Part model, mm, in its own coordinate system. A direction names the side the tool comes from. Coordinates: 2 decimals unless noted, no trailing zeros. Loops run counter-clockwise (first coordinate to the right, second up) from the corner with the lowest first, then second, coordinate; pieces in that order, holes last. Notation, with made-up numbers: (87.25, 12) -> (131.25, 12) arc R22 cw to (131.25, 21) -> close; hole circle Ø8 at (-16, 66). An arc over 180 degrees is marked (long way). One line per item, written item: value. Start each with the question number.
from build123d import *

# Parameters (mm, degrees)
F0_W     = 5.9
F0_H     = 0.3
F1_DEPTH = 2.5
F0_H_2   = 3.125
F2_DEPTH = 0.2
F4_DEPTH = 6.501


with BuildPart() as f1:
    # F0 (on Front) → F1 (new body)
    with BuildSketch(Plane.XZ):
        Polygon((-3.25, 16.5), (-3.25, 0), (-2.95, 0), (-2.95, 1), (-2.95, 1.3), (-2.95, 4.425), (-2.95, 4.725), (-2.95, 7.85), (-2.95, 8.15), (-2.95, 11.275), (-2.95, 11.575), (-2.95, 14.7), (-2.95, 15), (-2.95, 16.5), align=None)
        Polygon((2.95, 1), (2.95, 0), (3.25, 0), (3.25, 16.5), (2.95, 16.5), (2.95, 15), (2.95, 14.7), (2.95, 11.575), (2.95, 11.275), (2.95, 8.15), (2.95, 7.85), (2.95, 4.725), (2.95, 4.425), (2.95, 1.3), align=None)
        with Locations((0, 14.85)):
            Rectangle(F0_W, F0_H)
        with Locations((0, 11.425)):
            Rectangle(F0_W, F0_H)
        with Locations((0, 8)):
            Rectangle(F0_W, F0_H)
        with Locations((0, 4.575)):
            Rectangle(F0_W, F0_H)
        with Locations((0, 1.15)):
            Rectangle(F0_W, F0_H)
    extrude(amount=F1_DEPTH)

    # F0 (on Front) → F2 (join)
    with BuildSketch(Plane.XZ):
        with Locations((0, 13.1375)):
            Rectangle(F0_W, F0_H_2)
        with Locations((0, 6.2875)):
            Rectangle(F0_W, F0_H_2)
    extrude(amount=F2_DEPTH)

    # F3 (on face) → F4 (cut, through all)
    with BuildSketch(Plane.YZ.offset(3.25)):
        Polygon((-1.9, 0), (-0.6, 0), (-0.6, 1), (-1.25, 1), align=None)
    extrude(amount=-F4_DEPTH, mode=Mode.SUBTRACT)


solid = f1.part
1) Pull direction X, two halves, no side cores. Call faces 6 (the flat face through (-3.25, -1, 8)), 7 (the flat face through (-3, -2.5, 8)), 8 (the flat face through (0, -1, 4.725)): +X half, -X half, draft (parallel to the pull), parting line (faces both ways), or undercut.
2) Probe line 1 (Z direction, x = 2.5, y = -0.9) (3 decimals); line 2 (X direction, y = -1.2, z = 13.25); line 3 (Y direction, x = 2.75, z = 12). List the from-to ranges inside material, lowest first. Write a range as from..to.
3) Slice it at D-D (y = -1.55). Give the cut face in (x, z) (3 decimals).
4) Slice it at C-C (y = -0.4). Give the cut face in (x, z) (3 decimals).
5) Slice it at B-B (x = 1.5). Give the cut face in (y, z) (3 decimals).
6) Pin check, flat tips, straight feed: pin 1 Ø0.8 at (x, y) = (-1, -1) entering from -Z; pin 2 Ø0.8 at (x, y) = (1, -1.5) entering from +Z. Stop position of each tip, or through.
7) Tool access for faces 1 (the flat face through (2.95, -2, 0.5)), 2 (the flat face through (-2.95, -1, 3)), 3 (the flat face through (2.95, -1, 16)), 4 (the flat face through (3.25, -1, 8)), 5 (the flat face through (0, -0.2, 6)): list every direction of +Z, -Z, +X, -X, +Y, -Y with a clear straight run to the whole face (end or side of a thin tool).
8) Slice it at A-A (z = 15.5). Give the cut face in (x, y).
Check sheet entries:
1. face 6: -X half
1. face 7: draft
1. face 8: undercut
2. line 1: z = 1..1.3, 4.425..4.725, 7.85..8.15, 11.275..11.575, 14.7..15
2. line 2: x = -3.25..-2.95, 2.95..3.25
2. line 3: y = -0.2..0
3. outline: (-3.25, 0.538) -> (-2.95, 0.538) -> (-2.95, 1) -> (2.95, 1) -> (2.95, 0.538) -> (3.25, 0.538) -> (3.25, 16.5) -> (2.95, 16.5) -> (2.95, 15) -> (-2.95, 15) -> (-2.95, 16.5) -> (-3.25, 16.5) -> close; hole (-2.95, 1.3) -> (2.95, 1.3) -> (2.95, 4.425) -> (-2.95, 4.425) -> close; hole (-2.95, 4.725) -> (2.95, 4.725) -> (2.95, 7.85) -> (-2.95, 7.85) -> close; hole (-2.95, 8.15) -> (2.95, 8.15) -> (2.95, 11.275) -> (-2.95, 11.275) -> close; hole (-2.95, 11.575) -> (2.95, 11.575) -> (2.95, 14.7) -> (-2.95, 14.7) -> close
4. outline: (-3.25, 0) -> (-2.95, 0) -> (-2.95, 1) -> (2.95, 1) -> (2.95, 0) -> (3.25, 0) -> (3.25, 16.5) -> (2.95, 16.5) -> (2.95, 15) -> (-2.95, 15) -> (-2.95, 16.5) -> (-3.25, 16.5) -> close; hole (-2.95, 1.3) -> (2.95, 1.3) -> (2.95, 4.425) -> (-2.95, 4.425) -> close; hole (-2.95, 4.725) -> (2.95, 4.725) -> (2.95, 7.85) -> (-2.95, 7.85) -> close; hole (-2.95, 8.15) -> (2.95, 8.15) -> (2.95, 11.275) -> (-2.95, 11.275) -> close; hole (-2.95, 11.575) -> (2.95, 11.575) -> (2.95, 14.7) -> (-2.95, 14.7) -> close
5. outline: (-2.5, 1) -> (0, 1) -> (0, 1.3) -> (-2.5, 1.3) -> close; (-2.5, 4.425) -> (0, 4.425) -> (0, 8.15) -> (-2.5, 8.15) -> (-2.5, 7.85) -> (-0.2, 7.85) -> (-0.2, 4.725) -> (-2.5, 4.725) -> close; (-2.5, 11.275) -> (0, 11.275) -> (0, 15) -> (-2.5, 15) -> (-2.5, 14.7) -> (-0.2, 14.7) -> (-0.2, 11.575) -> (-2.5, 11.575) -> close
6. pin 1: stops at z = 1
6. pin 2: stops at z = 15
7. face 1: -Z, +Y, -Y
7. face 2: +Y, -Y
7. face 3: +Z, +Y, -Y
7. face 4: +Z, -Z, +X, +Y, -Y
7. face 5: -Y
8. outline: (-3.25, -2.5) -> (-2.95, -2.5) -> (-2.95, 0) -> (-3.25, 0) -> close; (2.95, -2.5) -> (3.25, -2.5) -> (3.25, 0) -> (2.95, 0) -> close
